Could you check a few things on this model? Use its own coordinates, in mm. Face numbers are marked on the shaded views. A direction names the side the tool comes from. Coordinates: 2 decimals unless noted, no trailing zeros. Write each loop counter-clockwise with the first axis right and the second up, starting at its lowest first coordinate (ties: lowest second). Pieces come first, ordered by that corner, then holes. Notation, with made-up numbers: (58, 48.5) - (64, 48.5) arc R12 ccw to (64, 69.5) - close; hole circle Ø7 at (-39.5, 58). An arc over 180 degrees is marked (long way). Answer as a JSON object with one key per item and string values. Group by question number.
1) Will these pins go through, and if not, where does the flat tip stop? pin 1 Ø1.5 at (x, z) = (12, 2) entering from +Y (3 decimals); pin 2 Ø2 at (x, z) = (18.5, -40.5) entering from +Y; pin 3 Ø4 at (y, z) = (2, -50.5) entering from -X; pin 4 Ø13 at (x, y) = (8.5, 13) entering from +Z.
2) If we section it at C-C (z = -31.4): Write out the boundary of the cut face in (x, y).
3) If we section it at D-D (y = 24): Write out the boundary of the cut face in (x, z), plus the area to 3 significant figures.
4) Please list where these lines run through material, in increasing order: line 1 along X through (y, z) = (13.5, -31.4); line 2 along X through (y, z) = (9.15, 2.45); line 3 along Y through (x, z) = (10.5, -31).
5) If we section it at B-B (x = 11.1): Write out the boundary of the cut face in (y, z) (3 decimals), plus the area to 3 significant figures.
6) If we section it at A-A (z = 2.45): Write out the boundary of the cut face in (x, y) (3 decimals), plus the area to 4 significant figures.
7) On a 3-axis mill with a long thin cutter (end or side, diameter ignored), from which of +Z, -Z, +X, -X, +Y, -Y can I reach the whole of each face in a straight line? I mean the marked faces 1, 2 and 3. Say none if no direction works.
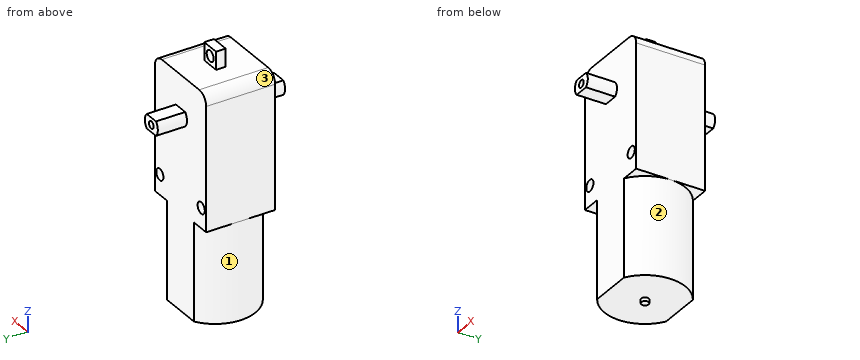
```python
from build123d import *

# Parameters (mm, degrees)
SKETCH1_W           = 22.2
SKETCH1_H           = 18.9
BOSS_EXTRUDE1_DEPTH = 36.9
SKETCH2_W           = 5.1
SKETCH2_H           = 2.65
BOSS_EXTRUDE2_DEPTH = 4.9
BOSS_EXTRUDE3_DEPTH = 26.71
SKETCH4_R           = 1
BOSS_EXTRUDE4_DEPTH = 1
BOSS_EXTRUDE5_DEPTH = 8
BOSS_EXTRUDE6_START = 8
BOSS_EXTRUDE6_DEPTH = 8
SKETCH8_R           = 1.5
CUT_EXTRUDE1_DEPTH  = 71.850495588
SKETCH9_R           = 1
CUT_EXTRUDE2_DEPTH  = 77.715722639
SKETCH10_R          = 1.56
CUT_EXTRUDE3_DEPTH  = 74.422762819
FILLET1_R           = 3


with BuildPart() as part:
    # Sketch1 → Boss-Extrude1 (new body)
    with BuildSketch(Plane.XY):
        with Locations((11.1, 9.45)):
            Rectangle(SKETCH1_W, SKETCH1_H)
    extrude(amount=-BOSS_EXTRUDE1_DEPTH)

    # Sketch2 → Boss-Extrude2 (add)
    with BuildSketch(Plane.XY):
        with Locations((11.1, 9.45)):
            Rectangle(SKETCH2_W, SKETCH2_H)
    extrude(amount=BOSS_EXTRUDE2_DEPTH)

    # Sketch3 → Boss-Extrude3 (add)
    with BuildSketch(Plane(origin=(0, 0, -36.9), x_dir=(-1, 0, 0), z_dir=(0, 0, -1))):
        with BuildLine():
            Line((-16.923014683, 18.9), (-5.276985317, 18.9))
            ThreePointArc((-5.276985317, 18.9), (0, 9.45), (-5.276985317, 0))
            Line((-5.276985317, 0), (-16.923014683, 0))
            ThreePointArc((-16.923014683, 0), (-22.2, 9.45), (-16.923014683, 18.9))
        make_face()
    extrude(amount=BOSS_EXTRUDE3_DEPTH)

    # Sketch4 → Boss-Extrude4 (add)
    with BuildSketch(Plane(origin=(0, 0, -63.61), x_dir=(-1, 0, 0), z_dir=(0, 0, -1))):
        with Locations((-11.1, 9.45)):
            Circle(SKETCH4_R)
    extrude(amount=BOSS_EXTRUDE4_DEPTH)

    # Sketch5 → Boss-Extrude5 (add)
    with BuildSketch(Plane(origin=(0, 18.9, 0), x_dir=(1, 0, 0), z_dir=(0, 1, 0))):
        with BuildLine():
            Line((9.09064687, 12.95), (13.10935313, 12.95))
            ThreePointArc((13.10935313, 12.95), (13.9, 11), (13.10935313, 9.05))
            Line((13.10935313, 9.05), (9.09064687, 9.05))
            ThreePointArc((9.09064687, 9.05), (8.3, 11), (9.09064687, 12.95))
        make_face()
    extrude(amount=BOSS_EXTRUDE5_DEPTH)

    # Sketch6 → Boss-Extrude6 (add)
    with BuildSketch(Plane.XZ.offset(BOSS_EXTRUDE6_START)):
        with BuildLine():
            Line((9.09064687, -9.05), (13.10935313, -9.05))
            ThreePointArc((13.10935313, -9.05), (13.9, -11), (13.10935313, -12.95))
            Line((13.10935313, -12.95), (9.09064687, -12.95))
            ThreePointArc((9.09064687, -12.95), (8.3, -11), (9.09064687, -9.05))
        make_face()
    extrude(amount=-BOSS_EXTRUDE6_DEPTH)

    # Sketch8 → Cut-Extrude1 (cut, through all)
    with BuildSketch(Plane(origin=(0, 10.775, 0), x_dir=(1, 0, 0), z_dir=(0, 1, 0))):
        with Locations(Location((11.1, -2.45, 0), (0, 0, 270))):
            Circle(SKETCH8_R)
    extrude(amount=-CUT_EXTRUDE1_DEPTH, mode=Mode.SUBTRACT)

    # Sketch9 → Cut-Extrude2 (cut, through all)
    with BuildSketch(Plane(origin=(0, 26.9, 0), x_dir=(1, 0, 0), z_dir=(0, 1, 0))):
        with Locations(Location((11.1, 11, 0), (0, 0, 270))):
            Circle(SKETCH9_R)
    extrude(amount=-CUT_EXTRUDE2_DEPTH, mode=Mode.SUBTRACT)

    # Sketch10 → Cut-Extrude3 (cut, through all)
    with BuildSketch(Plane(origin=(0, 18.9, 0), x_dir=(1, 0, 0), z_dir=(0, 1, 0))):
        with Locations(Location((2.14, 31.4, 0), (0, 0, 270))):
            Circle(SKETCH10_R)
        with Locations(Location((20.06, 31.4, 0), (0, 0, 270))):
            Circle(SKETCH10_R)
    extrude(amount=-CUT_EXTRUDE3_DEPTH, mode=Mode.SUBTRACT)

    # Fillet1
    fillet1_edges = [part.edges().sort_by_distance(p)[0] for p in [
        (22.2, 9.45, 0),
        (0, 9.45, 0),
    ]]
    fillet(fillet1_edges, radius=FILLET1_R)


solid = part.part
```
Here are the results:
{
 "1": {"pin 1": "stops at y = 10.775", "pin 2": "stops at y = 18.52", "pin 3": "stops at x = 1.43", "pin 4": "stops at z = 4.9"},
 "2": {"outline": "(0, 0) - (0.58, 0) - (0.58, 18.9) - (0, 18.9) - close; (3.7, 0) - (18.5, 0) - (18.5, 18.9) - (3.7, 18.9) - close; (21.62, 0) - (22.2, 0) - (22.2, 18.9) - (21.62, 18.9) - close"},
 "3": {"outline": "(9.09, -12.95) - (13.11, -12.95) arc R2.8 ccw to (13.11, -9.05) - (9.09, -9.05) arc R2.8 ccw to start; hole circle Ø2 at (11.1, -11)", "area": "16.8 mm²"},
 "4": {"line 1": "x = 0 to 0.58, 3.7 to 18.5, 21.62 to 22.2", "line 2": "x = 8.55 to 9.6, 12.6 to 13.65", "line 3": "y = 0 to 18.9"},
 "5": {"outline": "(-8, -12.95) - (0, -12.95) - (0, -63.61) - (8.45, -63.61) - (8.45, -64.61) - (10.45, -64.61) - (10.45, -63.61) - (18.9, -63.61) - (18.9, -12.95) - (26.9, -12.95) - (26.9, -12) - (-8, -12) - close; (-8, -10) - (26.9, -10) - (26.9, -9.05) - (18.9, -9.05) - (18.9, 0) - (10.775, 0) - (10.775, 0.95) - (8.125, 0.95) - (8.125, 0) - (0, 0) - (0, -9.05) - (-8, -9.05) - close; (8.125, 3.95) - (10.775, 3.95) - (10.775, 4.9) - (8.125, 4.9) - close", "area": "1,200 mm²"},
 "6": {"outline": "(8.55, 8.125) - (9.6, 8.125) - (9.6, 10.775) - (8.55, 10.775) - close; (12.6, 8.125) - (13.65, 8.125) - (13.65, 10.775) - (12.6, 10.775) - close", "area": "5.565 mm²"},
 "7": {"face 1": "-Z, -X", "face 2": "-Z, +X", "face 3": "+Z, -X, +Y, -Y"}
}
